The listing builds one solid part. Answer for the finished solid, in the listing's coordinates (mm). A direction names the side the tool comes from. Give positions to 0.01 mm unless a question says otherwise; leave off trailing zeros. Write each loop counter-clockwise with the first axis right and the second up, starting at its lowest first coordinate (ties: lowest second). Pieces come first, ordered by that corner, then holes. Notation, with made-up numbers: (-19, -21) - (-2, -21) arc R21 cw to (-2, -1) - close; hole circle Ø7 at (1.5, 74.5). An arc over 180 degrees is marked (long way). Use a Markdown table: item, result. Add a question column.
from build123d import *

# Parameters (mm, degrees)
SKETCH1_W           = 30
SKETCH1_H           = 45
SKETCH1_W_2         = 15
SKETCH1_H_2         = 50
BOSS_EXTRUDE3_DEPTH = 50
BOSS_EXTRUDE4_DEPTH = 175
BOSS_EXTRUDE6_DEPTH = 100


with BuildPart() as part:
    # Sketch1 → Boss-Extrude3 (new body)
    with BuildSketch(Plane(origin=(0, 0, 0), x_dir=(1, 0, 0), z_dir=(0, 1, 0))):
        Polygon((85, 87.5), (-85, 87.5), (-85, 37.5), (-70, 37.5), (-35, 37.5), (-35, 22.5), (-70, 22.5), (-70, -22.5), (-35, -22.5), (-35, -37.5), (-85, -37.5), (-85, -87.5), (85, -87.5), (85, -37.5), (35, -37.5), (35, -22.5), (70, -22.5), (70, 22.5), (35, 22.5), (35, 37.5), (70, 37.5), (85, 37.5), align=None)
        with Locations((-85, 0)):
            Rectangle(SKETCH1_W, SKETCH1_H)
        with Locations((-92.5, 62.5)):
            Rectangle(SKETCH1_W_2, SKETCH1_H_2)
        Polygon((-85, 37.5), (-100, 37.5), (-100, 22.5), (-70, 22.5), (-35, 22.5), (-35, 37.5), (-70, 37.5), align=None)
        Polygon((-70, -22.5), (-100, -22.5), (-100, -37.5), (-85, -37.5), (-35, -37.5), (-35, -22.5), align=None)
        with Locations((-92.5, -62.5)):
            Rectangle(SKETCH1_W_2, SKETCH1_H_2)
        with Locations((92.5, 62.5)):
            Rectangle(SKETCH1_W_2, SKETCH1_H_2)
        Polygon((100, 37.5), (85, 37.5), (70, 37.5), (35, 37.5), (35, 22.5), (70, 22.5), (100, 22.5), align=None)
        with Locations((85, 0)):
            Rectangle(SKETCH1_W, SKETCH1_H)
        Polygon((100, -37.5), (100, -22.5), (70, -22.5), (35, -22.5), (35, -37.5), (85, -37.5), align=None)
        with Locations((92.5, -62.5)):
            Rectangle(SKETCH1_W_2, SKETCH1_H_2)
    extrude(amount=BOSS_EXTRUDE3_DEPTH)

    # Sketch5 → Boss-Extrude4 (add)
    with BuildSketch(Plane.XY.offset(87.5)):
        Polygon((-100, 50), (-85, 50), (0, 125), (85, 50), (100, 50), (100, 0), (-100, 0), align=None)
    extrude(amount=-BOSS_EXTRUDE4_DEPTH)

    # Sketch18 → Boss-Extrude6 (add, symmetric)
    with BuildSketch(Plane(origin=(0, 0, 0), x_dir=(0, 0, -1), z_dir=(1, 0, 0))):
        Polygon((-87.5, 50), (-37.5, 50), (-37.5, 100), (-22.5, 100), (-22.5, 65), (22.5, 65), (22.5, 100), (37.5, 100), (37.5, 50), (87.5, 50), (87.5, 0), (-87.5, 0), align=None)
    extrude(amount=BOSS_EXTRUDE6_DEPTH, both=True)


solid = part.part
1. Consider L1, parallel to Z at x = 60, y = 86.5; L2, parallel to Y at x = -39, z = -23; L3, parallel to Z at x = 84, y = 53. Determine where each line is inside the solid, lowest interval first. Write a range as [from, to].
2. Which of the six approach directions +Z, -Z, +X, -X, +Y, -Y give full straight-line access (tool end or side, diameter ignored) to faces 1 (the flat face through (-64, 100, 30)), 2 (the flat face through (73, 81, -37.5)), 3 (the flat face through (73, 80, 37.5)), 4 (the flat face through (-72, 80, 37.5))?
3. The part is cut by section A-A (z = 17). Give the vertices of the cut face in (x, y), and give its area (3 significant figures).
4. The part is cut by section D-D (z = -41.5). Give the vertices of the cut face in (x, y), and give its area (3 significant figures).
5. The part is cut by section C-C (x = 64.5). Give the vertices of the cut face in (y, z).
6. For a pull along Z with two mould halves and no side action, classify faces 5 (the flat face through (73, 86, -22.5)), 6 (the flat face through (-64, 100, -30)), 7 (the flat face through (-72, 81, -37.5)) as released by +Z, released by -Z, zero draft, split by the parting line, or undercut.
7. Given P1, Ø7.5, axis at x = -50, z = -32, coming from the +Y side; P2, Ø16.5, axis at x = 94, z = 62.5, coming from the +Y side; P3, Ø16, axis at x = 85.5, z = -4, coming from the +Y side; P4, Ø17.5, axis at x = -53, y = 88.5, coming from the +Z side, each flat-ended and moving along its own axis, determine where each tip first touches the part or whether it passes through.
8. The part is cut by section B-B (y = 92). Give the vertices of the cut face in (x, z), and give its area (3 significant figures).
Check values:
| question | item | result |
|---|---|---|
| 1 | L1 | z = [-37.5, -22.5], [22.5, 37.5] |
| 1 | L2 | y = [0, 100] |
| 1 | L3 | z = [-37.5, 37.5] |
| 2 | face 1 | +Z, -Z, -X, +Y |
| 2 | face 2 | -Z, +X, +Y |
| 2 | face 3 | +Z, +X, +Y |
| 2 | face 4 | +Z, -X, +Y |
| 3 | outline | (-100, 0) - (100, 0) - (100, 65) - (68, 65) - (0, 125) - (-68, 65) - (-100, 65) - close |
| 3 | area | 17,100 mm2 |
| 4 | outline | (-100, 0) - (100, 0) - (100, 50) - (85, 50) - (0, 125) - (-85, 50) - (-100, 50) - close |
| 4 | area | 16,400 mm2 |
| 5 | outline | (0, -87.5) - (68.09, -87.5) - (68.09, -37.5) - (100, -37.5) - (100, -22.5) - (68.09, -22.5) - (68.09, 22.5) - (100, 22.5) - (100, 37.5) - (68.09, 37.5) - (68.09, 87.5) - (0, 87.5) - close |
| 6 | face 5 | undercut |
| 6 | face 6 | zero draft |
| 6 | face 7 | released by -Z |
| 7 | P1 | stops at y = 100 |
| 7 | P2 | stops at y = 50 |
| 7 | P3 | stops at y = 65 |
| 7 | P4 | stops at z = 87.5 |
| 8 | outline | (-100, -37.5) - (-37.4, -37.5) - (-37.4, -87.5) - (37.4, -87.5) - (37.4, -37.5) - (100, -37.5) - (100, -22.5) - (37.4, -22.5) - (37.4, 22.5) - (100, 22.5) - (100, 37.5) - (37.4, 37.5) - (37.4, 87.5) - (-37.4, 87.5) - (-37.4, 37.5) - (-100, 37.5) - (-100, 22.5) - (-37.4, 22.5) - (-37.4, -22.5) - (-100, -22.5) - close |
| 8 | area | 16,800 mm2 |
